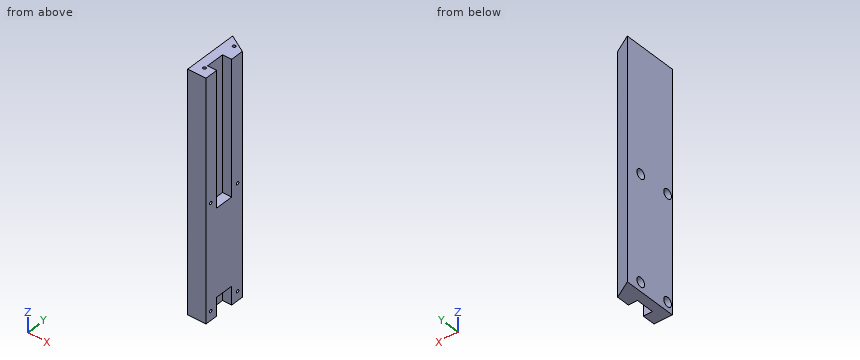
Autodesk Inventor part; units mm, degrees
ref_plane "YZ Plane" through (0, 0, 0) normal (1, 0, 0) x (0, 1, 0)
ref_plane "XZ Plane" through (0, 0, 0) normal (0, 1, 0) x (-1, 0, 0)
ref_plane "XY Plane" through (0, 0, 0) normal (0, 0, 1) x (1, 0, 0)
sketch "Sketch1" plane through (0, 0, 0) normal (0, 0, 1) x (1, 0, 0)
  line L0 (0, 0) -> (0, 76.2)
  line L1 (0, 76.2) -> (25.4, 61.5353)
  line L2 (25.4, 61.5353) -> (25.4, 0)
  line L3 (25.4, 0) -> (0, 0)
  dimension "d0" = 25.4
  dimension "d1" = 76.2
  dimension "d2" = 60
extrude "Extrusion1" add sketch "Sketch1" along normal blind 330.2
sketch "Sketch3" plane through (0, 0, 330.2) normal (0, 0, 1) x (1, 0, 0)
  line L0 (12.7, 43.4677) -> (25.4, 43.4677)
  line L1 (25.4, 43.4677) -> (25.4, 18.0677)
  line L2 (25.4, 18.0677) -> (12.7, 18.0677)
  line L3 (12.7, 18.0677) -> (12.7, 43.4677)
  line L4 (25.4, 0) -> (25.4, 61.5353)
  point P0 (0, 0)
  point P1 (25.4, 30.7677)
  dimension "d5" = 12.7
  dimension "d6" = 25.4
extrude "Extrusion2" cut sketch "Sketch3" against normal blind 185
sketch "Sketch4" plane through (0, 0, 0) normal (0, 0, -1) x (-1, 0, 0)
  line L0 (-12.7, 18.0677) -> (-12.7, 43.4677)
  line L1 (-12.7, 18.0677) -> (-12.7, 43.4677)
  line L2 (-25.4, 18.0677) -> (-12.7, 18.0677)
  line L3 (-25.4, 43.4677) -> (-25.4, 18.0677)
  line L4 (-12.7, 43.4677) -> (-25.4, 43.4677)
  point P0 (0, 0)
extrude "Extrusion3" cut sketch "Sketch4" against normal blind 25.4
sketch "Sketch5" plane through (25.4, 61.5353, 330.2) normal (1, 0, 0) x (0, 0, -1)
  line L0 (172.3, -53.5353) -> (317.5, -53.5353) construction
  line L1 (317.5, -53.5353) -> (317.5, -8) construction
  line L2 (317.5, -8) -> (172.3, -8) construction
  line L3 (172.3, -8) -> (172.3, -53.5353) construction
  line L4 (304.8, -18.0677) -> (304.8, -43.4677) construction
  line L5 (185, -18.0677) -> (185, -43.4677) construction
  line L6 (330.2, -61.5353) -> (0, -61.5353)
  circle A0 centre (172.3, -53.5353) radius 2
  circle A1 centre (172.3, -8) radius 2
  circle A2 centre (317.5, -8) radius 2
  circle A3 centre (317.5, -53.5353) radius 2
  point P0 (185, -30.7677)
  point P1 (172.3, -30.7677)
  point P2 (304.8, -30.7677)
  point P3 (317.5, -30.7677)
  dimension "d11" = 12.7
  dimension "d12" = 12.7
  dimension "d13" = 8
  dimension "d14" = 4
  dimension "d15" = 4
  dimension "d16" = 4
  dimension "d17" = 4
extrude "Extrusion4" cut sketch "Sketch5" against normal through all
sketch "Sketch6" plane through (0, 0, 0) normal (-1, 0, 0) x (0, 0, 1)
  circle A0 centre (157.9, 53.5353) radius 2
  circle A1 centre (157.9, 8) radius 2
  circle A2 centre (12.7, 8) radius 2
  circle A3 centre (12.7, 53.5353) radius 2
  circle A4 centre (157.9, 53.5353) radius 2
  circle A5 centre (157.9, 53.5353) radius 6.5
  circle A6 centre (157.9, 8) radius 2
  circle A7 centre (157.9, 8) radius 6.5
  circle A8 centre (12.7, 8) radius 2
  circle A9 centre (12.7, 8) radius 6.5
  circle A10 centre (12.7, 53.5353) radius 2
  circle A11 centre (12.7, 53.5353) radius 6.5
  point P0 (0, 0)
  dimension "d20" = 13
  dimension "d21" = 13
  dimension "d22" = 13
  dimension "d23" = 13
extrude "Extrusion5" cut sketch "Sketch6" against normal blind 12.7 contours A0 | A1 | A2 | A3 | A5 | A7 | A9 | A11
sketch "Sketch7" plane through (0, 0, 330.2) normal (0, 0, 1) x (1, 0, 0)
  circle A0 centre (12.7, 63.1) radius 2
  circle A1 centre (12.7, 13.1) radius 2
  line L0 (12.7, 63.1) -> (12.7, 13.1)
  line L1 (0, 76.2) -> (0, 0)
  line L2 (0, 0) -> (25.4, 0)
  point P0 (12.7, 38.1)
  point P1 (0, 38.1)
  point P2 (12.7, 0)
  dimension "d26" = 4
  dimension "d27" = 4
  dimension "d28" = 50
extrude "Extrusion6" cut sketch "Sketch7" against normal blind 38.1
properties part number "HB01" material "Polyethylene, High Density"
Can you work these out from the model? Positions are in its coordinate system, mm. Coordinates: 2 decimals unless noted, no trailing zeros. Write each loop counter-clockwise with the first axis right and the second up, starting at its lowest first coordinate (ties: lowest second). Pieces come first, ordered by that corner, then holes. Notation, with made-up numbers: (42, -26.75) -> (61, -26.75) arc R36 cw to (61, 9.25) -> close; hole circle Ø2 at (42.5, 35.5). An arc over 180 degrees is marked (long way). Write each question's results on one line, items separated by ' | '. Start each with the question number.
Item 1: If we section it at B-B, the plane z = 273: Write out the boundary of the cut face in (x, y), and give its area (3 significant figures).
Item 2: Please list where these lines run through material, in increasing order: probe 1 along Y at (x, z) = (4.25, 12.7); probe 2 along Z at (x, y) = (11.25, 13.5); probe 3 along Z at (x, y) = (5.25, 51.5).
Item 3: If we section it at C-C, the plane z = 80.5: Write out the boundary of the cut face in (x, y).
Item 4: I'm going to push flat-ended pins straight in: P1, Ø3, axis at x = 15.5, z = 124, coming from the +Y side; P2, Ø10.5, axis at y = 53.54, z = 12.7, coming from the -X side; P3, Ø10, axis at x = 21.5, y = 33, coming from the +Z side; P4, Ø2.5, axis at y = 53.54, z = 157.9, coming from the +X side. Where does each tip first touch, or does it pass through?
Item 5: If we section it at A-A, the plane x = 7.25: Write out the boundary of the cut face in (y, z), and give its area (3 significant figures).
Answer block:
1) outline: (0, 0) -> (25.4, 0) -> (25.4, 18.07) -> (12.7, 18.07) -> (12.7, 43.47) -> (25.4, 43.47) -> (25.4, 61.54) -> (0, 76.2) -> close | area: 1,430 mm²
2) probe 1: 0 to 1.5, 14.5 to 47.04, 60.04 to 73.75 | probe 2: 0 to 9.24, 16.16 to 154.44, 161.36 to 292.1 | probe 3: 0 to 6.53, 18.87 to 151.73, 164.07 to 330.2
3) outline: (0, 0) -> (25.4, 0) -> (25.4, 61.54) -> (0, 76.2) -> close
4) P1: y = 68.12 | P2: x = 12.7 | P3: z = 145.2 | P4: through
5) outline: (0, 0) -> (72.01, 0) -> (72.01, 330.2) -> (0, 330.2) -> close; hole circle Ø13 at (8, 12.7); hole circle Ø13 at (8, 157.9); hole circle Ø13 at (53.54, 12.7); hole circle Ø13 at (53.54, 157.9) | area: 23,200 mm²
